from build123d import *

# Parameters (mm, degrees)
CHAMFER1_SIZE = 0.2


with BuildPart() as part:
    # Sketch1 → Revolve1 (revolve)
    with BuildSketch(Plane(origin=(0, 0, 0), x_dir=(0, 0, -1), z_dir=(1, 0, 0)), mode=Mode.PRIVATE) as revolve1_sk:
        Polygon((0, 3), (0, 7), (2, 7), (2, 5), (8, 5), (8, 3), align=None)
    revolve(revolve1_sk.sketch.rotate(Axis((0, 0, 0), (0, 0, -1)), 90), axis=Axis((0, 0, 0), (0, 0, -1)))

    # Chamfer1
    chamfer1_edges = [part.edges().sort_by_distance(p)[0] for p in [
        (-3, 0, -8),
        (-5, 0, -8),
        (-5, 0, -2),
        (-7, 0, -2),
        (-7, 0, 0),
        (-3, 0, 0),
    ]]
    chamfer(chamfer1_edges, length=CHAMFER1_SIZE)


solid = part.part
CAD build for the part. Positions are in the model's coordinates, mm. Coordinates: 2 decimals unless noted, no trailing zeros. Loops run counter-clockwise (first coordinate to the right, second up) from the corner with the lowest first, then second, coordinate; pieces in that order, holes last. Notation, with made-up numbers: (31, -34) - (67, -34) arc R17 ccw to (67, -15) - close; hole circle Ø5 at (52.25, -3). An arc over 180 degrees is marked (long way). Use one line per item in the form item = value. Start each with the question number.
1) Drill centre lines: L1, parallel to Y at x = 0, z = -6; L2, parallel to Y at x = -2, z = -7; L3, parallel to Z at x = 4.5, y = 5. Where is each one in solid material? Low to high. Write a range as from..to.
2) Two-plate mould, pull along X, no slides. Class faces 1 (the face through (3.23, 6.21, -1.01)), 2 (the face through (2.86, -0.9, -3.95)), 3 (the face through (-3, -2, 0)): +X half, -X half, draft (parallel to the pull), parting line (faces both ways), or undercut.
3) Band-saw the part on C-C (z = -6.75). Give the cut face in (x, y).
4) Flat gauge pins, fed straight in: pin 1 (1.5 mm diameter, centred on y = 2.5, z = -2, fed in from +X); pin 2 (1.5 mm diameter, centred on x = 0, z = -4, fed in from -Y); pin 3 (5.5 mm diameter, centred on x = 0, y = 0, fed in from +Z); pin 4 (1.5 mm diameter, centred on y = -3.5, z = -1, fed in from -X). Where does each tip first touch, or does it go through?
5) Band-saw the part on A-A (x = 0). Give the cut face in (y, z), and give its area (3 significant figures).
Check values:
q1.L1 = -5..-3, 3..5
q1.L2 = -4.58..-2.24, 2.24..4.58
q1.L3 = -2..0
q2.face_1 = parting line
q2.face_2 = undercut
q2.face_3 = draft
q3.outline = circle Ø10 at (0, 0); hole circle Ø6 at (0, 0)
q4.pin_1 = 6.77
q4.pin_2 = -5
q4.pin_3 = through
q4.pin_4 = -6.44
q5.outline = (-7, -1.8) - (-6.8, -2) - (-5.2, -2) - (-5, -2.2) - (-5, -7.8) - (-4.8, -8) - (-3.2, -8) - (-3, -7.8) - (-3, -0.2) - (-3.2, 0) - (-6.8, 0) - (-7, -0.2) - close; (3, -7.8) - (3.2, -8) - (4.8, -8) - (5, -7.8) - (5, -2.2) - (5.2, -2) - (6.8, -2) - (7, -1.8) - (7, -0.2) - (6.8, 0) - (3.2, 0) - (3, -0.2) - close
q5.area = 39.8 mm2
